Build history of the part. All positions in model axes, mm. A direction names the side the tool comes from. Round coordinates to 2 decimals unless told otherwise and drop trailing zeros. Write each loop counter-clockwise with the first axis right and the second up, starting at its lowest first coordinate (ties: lowest second). Pieces come first, ordered by that corner, then holes.
1) Saw through at B-B (y = 2.8). State how many separate pieces and enclosed holes the cut face has, plus the area to 3 significant figures.
2) Pull direction Z, two halves, no side cores. Call faces 4 (the flat face through (-6.5, 2, -32)), 5 (the flat face through (-12, 2, 29.13)), 6 (the cylindrical face through (3.63, 3.01, 20.83)): +Z half, -Z half, draft (parallel to the pull), parting line (faces both ways), or undercut.
3) Which spindle directions (+Z, -Z, +X, -X, +Y, -Y) get a long thin tool onto all of the face, cutting with end or side? Do faces 1 (the flat face through (-9.7, 2, 0)), 2 (the flat face through (-6.5, 2, 32)), 3 (the flat face through (9, 2, 29.13)). Say none if no direction does.
4) Flat gauge pins, fed straight in: pin 1 (1.5 mm diameter, centred on x = -11.5, y = 2, fed in from +Z); pin 2 (1.5 mm diameter, centred on x = 6.5, y = 1.5, fed in from -Z); pin 3 (2.5 mm diameter, centred on x = 2.43, z = 19.53, fed in from -Y); pin 4 (1.5 mm diameter, centred on y = 3, z = 31, fed in from +X). Where does each tip first touch, or does it go through?
5) Saw through at A-A (z = 19.53). Write the cut outline in (x, y).
6) Wall check: probe 1 along X at (y, z) = (3.65, 22.33); probe 2 along X at (y, z) = (1.1, 15.5); probe 3 along X at (y, z) = (3.3, 19.53). Give the ranges that are in metal, low to high.
7) Saw through at C-C (z = -12). Write the cut outline in (x, y), plus the area to 3 significant figures.
from build123d import *

# Parameters (mm, degrees)
SKETCH1_W            = 35.4
SKETCH1_H            = 58.26
SKETCH1_W_2          = 3.5
SKETCH1_H_2          = 49.5
BASE_DEPTH           = 4
SKETCH2_R            = 1.4
MOUNTING_ENDS_DEPTH  = 4
TOP_START            = -4
SKETCH3_R            = 1.5
SKETCH3_R_2          = 1
TOP_CUTOUTS_DEPTH    = 2
F_1MM_EDGE_FILLETS_R = 1


with BuildPart() as part:
    # Sketch1 → Base (new body)
    with BuildSketch(Plane(origin=(0, 0, 0), x_dir=(1, 0, 0), z_dir=(0, 1, 0))):
        Rectangle(SKETCH1_W, SKETCH1_H)
        with Locations((-11.45, 0)):
            Rectangle(SKETCH1_W_2, SKETCH1_H_2, mode=Mode.SUBTRACT)
        with Locations((11.45, 0)):
            Rectangle(SKETCH1_W_2, SKETCH1_H_2, mode=Mode.SUBTRACT)
    extrude(amount=BASE_DEPTH)

    # Sketch2 → Mounting Ends (add)
    # profile 1 of 2: a face of its own
    with BuildSketch(Plane(origin=(0, 0, 0), x_dir=(1, 0, 0), z_dir=(0, 1, 0))):
        with BuildLine():
            Line((-6.5, 29.13), (0.5, 29.13))
            Line((0.5, 29.13), (0.5, 33.13))
            ThreePointArc((0.5, 33.13), (-3, 36.63), (-6.5, 33.13))
            Line((-6.5, 33.13), (-6.5, 29.13))
        make_face()
        with Locations(Location((-3, 33, 0), (0, 0, 270))):
            Circle(SKETCH2_R, mode=Mode.SUBTRACT)
    # profile 2 of 2: a face of its own
    with BuildSketch(Plane(origin=(0, 0, 0), x_dir=(1, 0, 0), z_dir=(0, 1, 0))):
        with BuildLine():
            Line((-6.5, -29.13), (-6.5, -33.13))
            ThreePointArc((-6.5, -33.13), (-3, -36.63), (0.5, -33.13))
            Line((0.5, -33.13), (0.5, -29.13))
            Line((0.5, -29.13), (-6.5, -29.13))
        make_face()
        with Locations(Location((-3, -33, 0), (0, 0, 90))):
            Circle(SKETCH2_R, mode=Mode.SUBTRACT)
    extrude(amount=MOUNTING_ENDS_DEPTH)

    # Sketch3 → Top Cutouts (cut)
    with BuildSketch(Plane.XZ.offset(TOP_START)):
        with Locations(Location((-3.7, 22.33, 0), (0, 0, 90))):
            Circle(SKETCH3_R)
        with Locations(Location((-2.43, 19.53, 0), (0, 0, 90))):
            Circle(SKETCH3_R_2)
        with Locations(Location((2.43, 19.53, 0), (0, 0, 90))):
            Circle(SKETCH3_R_2)
        with Locations(Location((3.7, 22.33, 0), (0, 0, 90))):
            Circle(SKETCH3_R)
    extrude(amount=TOP_CUTOUTS_DEPTH, mode=Mode.SUBTRACT)

    # 1mm Edge Fillets
    f_1mm_edge_fillets_edges = [part.edges().sort_by_distance(p)[0] for p in [
        (-12.1, 0, -29.13),
        (-3, 0, -36.63),
        (0.5, 2, -29.13),
        (0.5, 0, -31.13),
        (-6.5, 2, -29.13),
        (-6.5, 0, -31.13),
        (-12.1, 0, 29.13),
        (-17.7, 0, 0),
        (9.1, 0, 29.13),
        (9.1, 0, -29.13),
        (-6.5, 2, 29.13),
        (-6.5, 0, 31.13),
        (0.5, 2, 29.13),
        (0.5, 0, 31.13),
        (-3, 0, 36.63),
        (17.7, 0, 0),
        (17.7, 2, 29.13),
        (-17.7, 2, 29.13),
        (-17.7, 2, -29.13),
        (17.7, 2, -29.13),
    ]]
    fillet(f_1mm_edge_fillets_edges, radius=F_1MM_EDGE_FILLETS_R)


solid = part.part
Evaluation:
1. separate pieces: 1
1. enclosed holes: 8
1. area: 1,780 mm2
2. face 4: draft
2. face 5: +Z half
2. face 6: undercut
3. face 1: +Y, -Y
3. face 2: +Z, -X, +Y, -Y
3. face 3: +Z, +X, +Y, -Y
4. pin 1: stops at z = 29.13
4. pin 2: stops at z = -29.13
4. pin 3: stops at y = 0
4. pin 4: stops at x = 0.5
5. outline: (-17.7, 1) arc R1 ccw to (-16.7, 0) - (-13.2, 0) - (-13.2, 4) - (-17.7, 4) - close; (-9.7, 0) - (9.7, 0) - (9.7, 4) - (3.43, 4) - (3.43, 2) - (1.43, 2) - (1.43, 4) - (-1.43, 4) - (-1.43, 2) - (-3.43, 2) - (-3.43, 4) - (-9.7, 4) - close; (13.2, 0) - (16.7, 0) arc R1 ccw to (17.7, 1) - (17.7, 4) - (13.2, 4) - close
6. probe 1: x = -17.7 to -13.2, -9.7 to -5.2, -2.2 to 2.2, 5.2 to 9.7, 13.2 to 17.7
6. probe 2: x = -17.7 to -13.2, -9.7 to 9.7, 13.2 to 17.7
6. probe 3: x = -17.7 to -13.2, -9.7 to -3.43, -1.43 to 1.43, 3.43 to 9.7, 13.2 to 17.7
7. outline: (-17.7, 1) arc R1 ccw to (-16.7, 0) - (-13.2, 0) - (-13.2, 4) - (-17.7, 4) - close; (-9.7, 0) - (9.7, 0) - (9.7, 4) - (-9.7, 4) - close; (13.2, 0) - (16.7, 0) arc R1 ccw to (17.7, 1) - (17.7, 4) - (13.2, 4) - close
7. area: 113 mm2
